Can you work these out from the drawing? Everything is in mm from the part's minimum corner. A direction names the side the tool comes from. Round coordinates to 2 decimals unless told otherwise and drop trailing zeros. One line per item, written item: value.
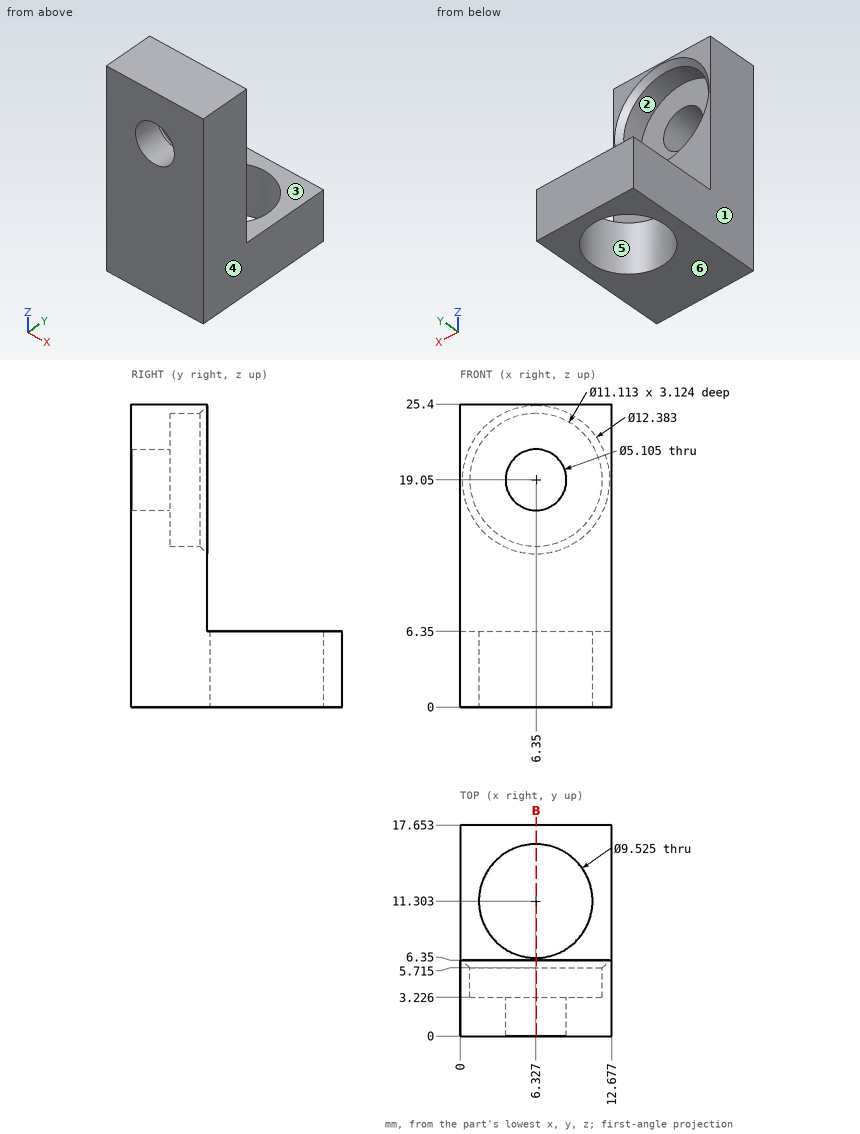
Q1. I want a section at B-B on x = 6.35. Give the number of separate pieces and of enclosed holes in the cut face, then the cut area to 3 significant figures.
Answers:
separate pieces: 3
enclosed holes: 0
area: 121 mm2
Q2. If we mould it in two halves opening along X, with no side actions, what happens to the marked faces 4, 5 and 6? For each: pulls with the +X half, pulls with the -X half, needs draft (parallel to the pull), parting line crosses it, or undercut.
Answers:
face 4: pulls with the +X half
face 5: undercut
face 6: needs draft
Q3. Which directions (+Z, -Z, +X, -X, +Y, -Y) give clear straight access to the entire face, cutting with the end or side of a thin tool? Please do the marked faces 1, 2 and 3.
Answers:
face 1: +Z, -Z, -X, +Y, -Y
face 2: +Y
face 3: +Z, +X, -X, +Y
Q4. For P1, Ø3, axis at x = 8, z = 13, coming from the +Y side; P2, Ø5.5, axis at x = 8, z = 21, coming from the +Y side, each with a flat end and sliding along its axis, tell me the tip position at first contact or that it passes through.
Answers:
P1: y = 6.35
P2: y = 3.23
Q5. I need wall thicknesses on line 1 along X through (y, z) = (3.9, 19.05); line 2 along X through (y, z) = (2, 19.05); line 3 along Z through (x, y) = (12, 13.5). Which ranges of each line are inside material? Lowest first, please.
Answers:
line 1: 0 to 0.79, 11.91 to 12.68
line 2: 0 to 3.8, 8.9 to 12.68
line 3: 0 to 6.35
